Could you check a few things on this model? Use its own coordinates, in mm. A direction names the side the tool comes from. Round coordinates to 2 decimals unless told otherwise and drop trailing zeros. Loops run counter-clockwise (first coordinate to the right, second up) from the corner with the lowest first, then second, coordinate; pieces in that order, holes last. Notation, with made-up numbers: (-7, 20) - (4, 20) arc R31 cw to (4, 55) - close; hole circle Ø3 at (-1, -17). An arc over 180 degrees is marked (long way). Use one line per item in the form item = value.
```python
from build123d import *

# Parameters (mm, degrees)
F0_W     = 449.58
F0_H     = 176.784
F1_DEPTH = 70.866
F3_DEPTH = 12.7
F6_W     = 263.13141
F6_H     = 176.784
F7_DEPTH = 76.2
F9_DEPTH = 189.485


with BuildPart() as f1:
    # F0 (on Top) → F1 (new body)
    with BuildSketch(Plane.XY):
        with Locations((4.088245, -16.670767)):
            Rectangle(F0_W, F0_H)
    extrude(amount=F1_DEPTH)

    # F2 (on face) → F3 (join, symmetric)
    with BuildSketch(Plane.XZ.offset(105.062767)):
        with BuildLine():
            Line((-169.266755, 0), (-99.416755, 0))
            ThreePointArc((-99.416755, 0), (-134.341755, 34.925), (-169.266755, 0))
        make_face()
        with BuildLine():
            ThreePointArc((-169.266755, 0), (-134.341755, -34.925), (-99.416755, 0))
            Line((-99.416755, 0), (-169.266755, 0))
        make_face()
        with BuildLine():
            ThreePointArc((162.203245, 0), (127.278245, 34.925), (92.353245, 0))
            Line((92.353245, 0), (162.203245, 0))
        make_face()
        with BuildLine():
            Line((162.203245, 0), (92.353245, 0))
            ThreePointArc((92.353245, 0), (127.278245, -34.925), (162.203245, 0))
        make_face()
    extrude(amount=F3_DEPTH, both=True)

    # F5: F1 across plane


with BuildPart() as f1_1:
    add(f1.part)
    add(f1.part.mirror(Plane(origin=(5.13005, -16.670767, 38.250844), x_dir=(1, 0, 0), z_dir=(0, -1, 0))))

    # F6 (on face) → F7 (join)
    with BuildSketch(Plane.XY.offset(70.866)):
        with Locations((-2.902493, -16.670767)):
            Rectangle(F6_W, F6_H)
    extrude(amount=F7_DEPTH)

    # F8 (on face) → F9 (cut, through all)
    with BuildSketch(Plane.XZ.offset(105.062767)):
        Polygon((-134.468198, 147.066), (-134.468198, 70.866), (-99.416755, 147.066), align=None)
        Polygon((128.663212, 147.066), (92.353245, 147.066), (128.663212, 70.866), align=None)
    extrude(amount=-F9_DEPTH, mode=Mode.SUBTRACT)


solid = f1_1.part
```
1. On a 3-axis mill with a long thin cutter (end or side, diameter ignored), from which of +Z, -Z, +X, -X, +Y, -Y can I reach the whole of each face in a straight line? I mean faces 1 (the face through (-129.8, 74.72, -34.63)), 2 (the face through (127, -92.363, -13)), 3 (the face through (178, -15, 70.866)). Say none if no direction works.
Solution:
face_1 = +Y
face_2 = -Z, +X, -X
face_3 = +Z, +X, +Y, -Y
2. If we section it at C-C, the plane z = 18.5: Write out the boundary of the cut face in (x, y).
Solution:
outline = (-220.7, -105.06) - (-163.96, -105.06) - (-163.96, -117.76) - (-104.72, -117.76) - (-104.72, -105.06) - (97.66, -105.06) - (97.66, -117.76) - (156.9, -117.76) - (156.9, -105.06) - (228.88, -105.06) - (228.88, 71.72) - (156.9, 71.72) - (156.9, 84.42) - (97.66, 84.42) - (97.66, 71.72) - (-104.72, 71.72) - (-104.72, 84.42) - (-163.96, 84.42) - (-163.96, 71.72) - (-220.7, 71.72) - close
3. For P1, Ø10, axis at x = 157.5, y = -1, coming from the +Z side; P2, Ø1.5, axis at x = -51, z = 95.5, coming from the +Y side; P3, Ø10, axis at x = -11, z = 37.5, coming from the -Y side, each with a flat end and sliding along its axis, tell me the tip position at first contact or that it passes through.
Solution:
P1 = 70.87
P2 = 71.72
P3 = -105.06
4. If we section it at D-D, the plane x = -77: Write out the boundary of the cut face in (y, z).
Solution:
outline = (-105.06, 0) - (71.72, 0) - (71.72, 147.07) - (-105.06, 147.07) - close
5. If we section it at A-A, the plane y = 44.5: Write out the boundary of the cut face in (x, z).
Solution:
outline = (-220.7, 0) - (228.88, 0) - (228.88, 70.87) - (128.66, 70.87) - (92.35, 147.07) - (-99.42, 147.07) - (-134.47, 70.87) - (-220.7, 70.87) - close
6. Please list where these lines run through material, in increasing order: line 1 along Y through (x, z) = (108, -26); line 2 along Z through (x, y) = (129.5, -5); line 3 along Z through (x, y) = (-61.5, -5).
Solution:
line_1 = -117.76 to -92.36, 59.02 to 84.42
line_2 = 0 to 70.87
line_3 = 0 to 147.07
7. If we section it at B-B, the plane z = -6.5: Write out the boundary of the cut face in (x, y), plus the area to 3 significant figures.
Solution:
outline = (-168.66, -117.76) - (-100.03, -117.76) - (-100.03, -92.36) - (-168.66, -92.36) - close; (-168.66, 59.02) - (-100.03, 59.02) - (-100.03, 84.42) - (-168.66, 84.42) - close; (92.96, -117.76) - (161.59, -117.76) - (161.59, -92.36) - (92.96, -92.36) - close; (92.96, 59.02) - (161.59, 59.02) - (161.59, 84.42) - (92.96, 84.42) - close
area = 6,970 mm^2
8. We'd pull the mould along X, two halves only. Please class faces 4 (the face through (1, -105.063, 73)), 5 (the face through (127, 84.421, 0)), 6 (the face through (228.878, -18, 35)): +X half, -X half, draft (parallel to the pull), parting line (faces both ways), or undercut.
Solution:
face_4 = undercut
face_5 = draft
face_6 = +X half
